Verification items for the finished model (mm, model axes). A direction names the side the tool comes from. Coordinates: 2 decimals unless noted, no trailing zeros. Loops run counter-clockwise (first coordinate to the right, second up) from the corner with the lowest first, then second, coordinate; pieces in that order, holes last.
Q1. Sectioned sample at D-D (z = 150). Enter the section's corners in (x, y), then the cut area to 3 significant figures.
Q2. Go/stop test with flat-tipped pins: P1, Ø4, axis at x = -12, z = 135, coming from the -Y side; P2, Ø5, axis at x = -116, y = -20.5, coming from the -Z side; P3, Ø12, axis at y = -33.5, z = 87.5, coming from the -X side. Record where each tip stops, or that it passes through.
Q3. Material ranges on probe 1 along X at (y, z) = (28, 171.45); probe 2 along Z at (x, y) = (-76, 36); probe 3 along Z at (x, y) = (38.1, 31.5) (3 decimals), recorded low to high.
Q4. Sectioned sample at B-B (z = 82.55). Enter the section's corners in (x, y) (3 decimals).
Q5. Access from +Z, -Z, +X, -X, +Y, -Y to the whole of each face (thin tool, end or side, straight path). Record for faces 4 (the face through (49.18, -12.17, 47.07)), 5 (the face through (-173, -12.7, 186)), 6 (the face through (91.26, -32.02, -27.95)), 7 (the face through (137.092, -0.178, 170.809)).
Q6. Mould release check, pull along Y, two halves, no side actions. Record for faces 1 (the face through (205.634, -32.017, 162.448)), 2 (the face through (-1, -50.8, 43)), 3 (the face through (-137.126, 0.178, 169.726)): +Y half, -Y half, draft (parallel to the pull), parting line (faces both ways), or undercut.
Q7. Sectioned sample at A-A (x = -76.2). Enter the section's corners in (y, z), then the cut area to 3 significant figures.
Q8. Sectioned sample at C-C (z = 180). Count the separate pieces of the cut face and the enclosed holes in it, then the cut area to 3 significant figures.
```python
from build123d import *

# Parameters (mm, degrees)
F1_DEPTH = 50.8
F3_DEPTH = 76.2
F4_R     = 38.1
F5_DEPTH = 12.7
F6_R     = 9.525
F7_DEPTH = 25.401
F8_R     = 19.05


with BuildPart() as f1:
    # F0 (on Front) → F1 (new body, symmetric)
    with BuildSketch(Plane.XZ):
        with BuildLine():
            ThreePointArc((-143.4367036526, 171.45), (-152.7360633499, 193.9006403027), (-175.1867036526, 203.2))
            ThreePointArc((-175.1867036526, 203.2), (-205.8548486372, 163.232495318), (-159.3117036526, 143.9536934298))
            ThreePointArc((-159.3117036526, 143.9536934298), (-147.6903970824, 155.575), (-143.4367036526, 171.45))
        make_face()
        with BuildLine():
            ThreePointArc((-162.4867036526, 171.45), (-164.1881810245, 165.1), (-168.8367036526, 160.4514773719))
            ThreePointArc((-168.8367036526, 160.4514773719), (-186.1852262806, 177.8), (-162.4867036526, 171.45))
        make_face(mode=Mode.SUBTRACT)
        with BuildLine():
            Line((92.075, 27.4963065702), (159.3117036526, 143.9536934298))
            ThreePointArc((159.3117036526, 143.9536934298), (144.5185586679, 179.667504682), (175.1867036526, 203.2))
            Line((175.1867036526, 203.2), (-175.1867036526, 203.2))
            ThreePointArc((-175.1867036526, 203.2), (-152.7360633499, 193.9006403027), (-143.4367036526, 171.45))
            ThreePointArc((-143.4367036526, 171.45), (-147.6903970824, 155.575), (-159.3117036526, 143.9536934298))
            Line((-159.3117036526, 143.9536934298), (-92.075, 27.4963065702))
            ThreePointArc((-92.075, 27.4963065702), (-60.325, 27.4963065702), (-44.45, 0))
            Line((-44.45, 0), (44.45, 0))
            ThreePointArc((44.45, 0), (60.325, 27.4963065702), (92.075, 27.4963065702))
        make_face()
        with BuildLine():
            ThreePointArc((175.1867036526, 203.2), (144.5185586679, 179.667504682), (159.3117036526, 143.9536934298))
            ThreePointArc((159.3117036526, 143.9536934298), (191.0617036526, 143.9536934298), (206.9367036526, 171.45))
            ThreePointArc((206.9367036526, 171.45), (197.6373439552, 193.9006403027), (175.1867036526, 203.2))
        make_face()
        with BuildLine():
            ThreePointArc((187.8867036526, 171.45), (181.5367036526, 160.4514773719), (168.8367036526, 160.4514773719))
            ThreePointArc((168.8367036526, 160.4514773719), (168.8367036526, 182.4485226281), (187.8867036526, 171.45))
        make_face(mode=Mode.SUBTRACT)
        with BuildLine():
            ThreePointArc((107.95, 0), (103.6963065702, 15.875), (92.075, 27.4963065702))
            Line((92.075, 27.4963065702), (82.55, 10.9985226281))
            ThreePointArc((82.55, 10.9985226281), (87.1985226281, 6.35), (88.9, 0))
            ThreePointArc((88.9, 0), (76.2, -12.7), (63.5, 0))
            Line((63.5, 0), (44.45, 0))
            ThreePointArc((44.45, 0), (76.2, -31.75), (107.95, 0))
        make_face()
        with BuildLine():
            Line((82.55, 10.9985226281), (92.075, 27.4963065702))
            ThreePointArc((92.075, 27.4963065702), (60.325, 27.4963065702), (44.45, 0))
            Line((44.45, 0), (63.5, 0))
            ThreePointArc((63.5, 0), (69.85, 10.9985226281), (82.55, 10.9985226281))
        make_face()
        with BuildLine():
            Line((-63.5, 0), (-44.45, 0))
            ThreePointArc((-44.45, 0), (-60.325, 27.4963065702), (-92.075, 27.4963065702))
            Line((-92.075, 27.4963065702), (-82.55, 10.9985226281))
            ThreePointArc((-82.55, 10.9985226281), (-69.85, 10.9985226281), (-63.5, 0))
        make_face()
        with BuildLine():
            ThreePointArc((-92.075, 27.4963065702), (-92.075, -27.4963065702), (-44.45, 0))
            Line((-44.45, 0), (-63.5, 0))
            ThreePointArc((-63.5, 0), (-82.55, -10.9985226281), (-82.55, 10.9985226281))
            Line((-82.55, 10.9985226281), (-92.075, 27.4963065702))
        make_face()
    extrude(amount=F1_DEPTH, both=True)

    # F2 (on face) → F3 (cut)
    with BuildSketch(Plane.XZ.offset(50.8)):
        Polygon((-50.5367805345, 44.45), (0, 44.45), (50.5367805345, 44.45), (142.1911357684, 203.2), (-142.1911357684, 203.2), align=None)
    extrude(amount=-F3_DEPTH, mode=Mode.SUBTRACT)

    # F4 (on Front) → F5 (cut, symmetric)
    with BuildSketch(Plane.XZ):
        with Locations((-175.1867036526, 171.45)):
            Circle(F4_R)
        with Locations((-76.2, 0)):
            Circle(F4_R)
        with Locations((76.2, 0)):
            Circle(F4_R)
        with Locations((175.1867036526, 171.45)):
            Circle(F4_R)
    extrude(amount=F5_DEPTH, both=True, mode=Mode.SUBTRACT)

    # F6 (on face) → F7 (cut, through all)
    with BuildSketch(Plane.XZ.offset(-25.4)):
        with Locations((38.1, 82.55)):
            Circle(F6_R)
        with Locations((-38.1, 82.55)):
            Circle(F6_R)
    extrude(amount=-F7_DEPTH, mode=Mode.SUBTRACT)

    # F8
    f8_edges = [f1.edges().sort_by_distance(p)[0] for p in [
        (-50.536781, -12.7, 44.45),
        (50.536781, -12.7, 44.45),
    ]]
    fillet(f8_edges, radius=F8_R)


solid = f1.part
```
Geometry check:
1. outline: (-198.6, -50.8) - (-111.48, -50.8) - (-111.48, 25.4) - (111.48, 25.4) - (111.48, -50.8) - (198.6, -50.8) - (198.6, -12.7) - (143.7, -12.7) - (143.7, 12.7) - (198.6, 12.7) - (198.6, 50.8) - (-198.6, 50.8) - (-198.6, 12.7) - (-143.7, 12.7) - (-143.7, -12.7) - (-198.6, -12.7) - close
1. area: 20,600 mm2
2. P1: stops at y = 25.4
2. P2: stops at z = 64.61
2. P3: stops at x = -130.18
3. probe 1: x = -206.94 to -187.89, -162.49 to 162.49, 187.89 to 206.94
3. probe 2: z = -31.75 to -12.7, 12.7 to 203.2
3. probe 3: z = 0 to 73.025, 92.075 to 203.2
4. outline: (-123.86, -50.8) - (-72.534, -50.8) - (-72.534, 25.4) - (-47.625, 25.4) - (-47.625, 50.8) - (-123.86, 50.8) - close; (-28.575, 25.4) - (28.575, 25.4) - (28.575, 50.8) - (-28.575, 50.8) - close; (47.625, 25.4) - (72.534, 25.4) - (72.534, -50.8) - (123.86, -50.8) - (123.86, 50.8) - (47.625, 50.8) - close
5. face 4: +Z, -Y
5. face 5: -X
5. face 6: +Y, -Y
5. face 7: +X
6. face 1: draft
6. face 2: -Y half
6. face 3: undercut
7. outline: (-50.8, -31.75) - (-12.7, -31.75) - (-12.7, -12.7) - (-50.8, -12.7) - close; (-50.8, 12.7) - (-12.7, 12.7) - (-12.7, 38.1) - (12.7, 38.1) - (12.7, 12.7) - (50.8, 12.7) - (50.8, 203.2) - (25.4, 203.2) - (25.4, 88.9) - (-50.8, 88.9) - close; (12.7, -31.75) - (50.8, -31.75) - (50.8, -12.7) - (12.7, -12.7) - close
7. area: 11,500 mm2
8. separate pieces: 5
8. enclosed holes: 0
8. area: 15,900 mm2
